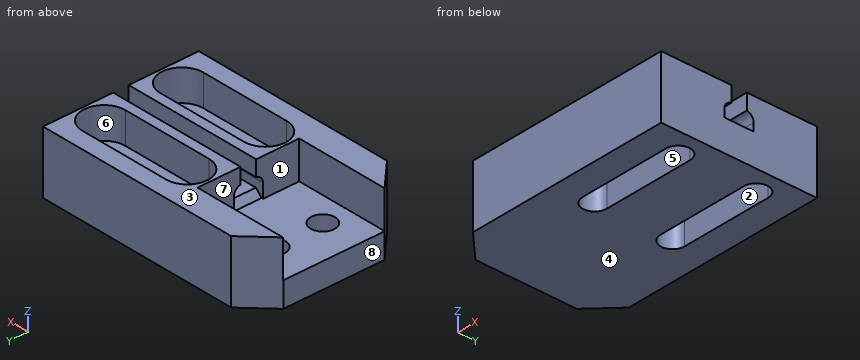
```python
from build123d import *

# Parameters (mm, degrees)
PROFILESKETCH3_W                           = 30
PROFILESKETCH3_H                           = 20
PROFILEBOSS_EXTRUDE1_DEPTH                 = 8
MICROSWITCHCUTSKETCH4_W                    = 12.05
MICROSWITCHCUTSKETCH4_H                    = 13.05
MICROSWITCHCUT_EXTRUDE1_DEPTH              = 4.8
SKETCH5_R                                  = 1.55
MICROSWITCHMOUNTINGHOLESCUT_EXTRUDE2_DEPTH = 3.1
SMALLCHANNELCABLESKETCH6_W                 = 17.95
SMALLCHANNELCABLESKETCH6_H                 = 2
SMALLCHANNELCABLECUT_EXTRUDE3_DEPTH        = 2
LARGECHANNELCABLESKETCH7_W                 = 17.95
LARGECHANNELCABLESKETCH7_H                 = 3.75
LARGECHANNELCABLECUT_EXTRUDE4_DEPTH        = 2
CHAMFER1_SIZE                              = 1
MOUNTSLOTBORECUT_EXTRUDE1_DEPTH            = 4
CHAMFER2_SIZE                              = 3.5
FILLET3_R                                  = 1


with BuildPart() as part:
    # ProfileSketch3 → ProfileBoss-Extrude1 (new body)
    with BuildSketch(Plane.XY):
        with Locations((15, 10)):
            Rectangle(PROFILESKETCH3_W, PROFILESKETCH3_H)
        with BuildLine():
            Line((15.15, 16.55), (26.9, 16.55))
            ThreePointArc((26.9, 16.55), (28.45, 15), (26.9, 13.45))
            Line((26.9, 13.45), (15.15, 13.45))
            ThreePointArc((15.15, 13.45), (13.6, 15), (15.15, 16.55))
        make_face(mode=Mode.SUBTRACT)
        with BuildLine():
            Line((15.15, 6.55), (26.9, 6.55))
            ThreePointArc((26.9, 6.55), (28.45, 5), (26.9, 3.45))
            Line((26.9, 3.45), (15.15, 3.45))
            ThreePointArc((15.15, 3.45), (13.6, 5), (15.15, 6.55))
        make_face(mode=Mode.SUBTRACT)
    extrude(amount=PROFILEBOSS_EXTRUDE1_DEPTH)

    # MicroSwitchCutSketch4 → MicroSwitchCut-Extrude1 (cut)
    with BuildSketch(Plane.XY.offset(8)):
        with Locations((6.025, 10)):
            Rectangle(MICROSWITCHCUTSKETCH4_W, MICROSWITCHCUTSKETCH4_H)
    extrude(amount=-MICROSWITCHCUT_EXTRUDE1_DEPTH, mode=Mode.SUBTRACT)

    # Sketch5 → MicroSwitchMountingHolesCut-Extrude2 (cut)
    with BuildSketch(Plane.XY.offset(3.2)):
        with Locations((5.05, 13.175)):
            Circle(SKETCH5_R)
        with Locations((5.05, 6.825)):
            Circle(SKETCH5_R)
    extrude(amount=-MICROSWITCHMOUNTINGHOLESCUT_EXTRUDE2_DEPTH, mode=Mode.SUBTRACT)

    # SmallChannelCableSketch6 → SmallChannelCableCut-Extrude3 (cut)
    with BuildSketch(Plane.XY.offset(8)):
        with Locations((21.025, 10)):
            Rectangle(SMALLCHANNELCABLESKETCH6_W, SMALLCHANNELCABLESKETCH6_H)
    extrude(amount=-SMALLCHANNELCABLECUT_EXTRUDE3_DEPTH, mode=Mode.SUBTRACT)

    # LargeChannelCableSketch7 → LargeChannelCableCut-Extrude4 (cut)
    with BuildSketch(Plane.XY.offset(6)):
        with Locations((21.025, 10)):
            Rectangle(LARGECHANNELCABLESKETCH7_W, LARGECHANNELCABLESKETCH7_H)
    extrude(amount=-LARGECHANNELCABLECUT_EXTRUDE4_DEPTH, mode=Mode.SUBTRACT)

    # Chamfer1
    # the kernel refuses this chamfer: 1 mm, written as the material it takes off along each edge
    with BuildSketch(Plane(origin=(12.05, 8.125, 4), x_dir=(0.9996219169112968, 0, 0.02749587661058651), z_dir=(0, 1, 0))) as chamfer1_piece_1_section:
        Polygon((CHAMFER1_SIZE * 0.999621916911, CHAMFER1_SIZE * 0.0274958766106), (-CHAMFER1_SIZE * 0.0274958766106, CHAMFER1_SIZE * 0.999621916911), (0, 0), align=None)
    chamfer1_piece_1 = extrude(amount=3.75, mode=Mode.PRIVATE)
    chamfer1_piece_1 = split(chamfer1_piece_1, bisect_by=Plane(origin=(12.395718412, 10, 3.2), z_dir=(0, 0, 1)), keep=Keep.TOP, mode=Mode.PRIVATE)
    add(chamfer1_piece_1, mode=Mode.SUBTRACT)

    # Sketch6 → MountSLotBoreCut-Extrude1 (cut)
    with BuildSketch(Plane.XY.offset(8)):
        with BuildLine():
            Line((15.15, 17.75), (26.9, 17.75))
            ThreePointArc((26.9, 17.75), (29.65, 15), (26.9, 12.25))
            Line((26.9, 12.25), (15.15, 12.25))
            ThreePointArc((15.15, 12.25), (12.4, 15), (15.15, 17.75))
        make_face()
        with BuildLine():
            Line((15.15, 7.75), (26.9, 7.75))
            ThreePointArc((26.9, 7.75), (29.65, 5), (26.9, 2.25))
            Line((26.9, 2.25), (15.15, 2.25))
            ThreePointArc((15.15, 2.25), (12.4, 5), (15.15, 7.75))
        make_face()
    extrude(amount=-MOUNTSLOTBORECUT_EXTRUDE1_DEPTH, mode=Mode.SUBTRACT)

    # Chamfer2
    chamfer2_edges = [part.edges().sort_by_distance(p)[0] for p in [
        (0, 20, 4),
        (0, 0, 4),
    ]]
    chamfer(chamfer2_edges, length=CHAMFER2_SIZE)

    # Fillet3
    # the kernel refuses this fillet: 1 mm, written as the material it adds along each edge
    with BuildSketch(Plane(origin=(12.05, 11.875, 6), x_dir=(0, 0, -1), z_dir=(1, 0, 0))) as fillet3_piece_1:
        with BuildLine():
            CenterArc((0.992156742, -1), FILLET3_R, 90, 82.819244219)
            Line((0, -0.875), (-0.019843135, -0.8725))
            ThreePointArc((-0.019843135, -0.8725), (-0.02, -0.4375), (-0.02, 0))
            Line((-0.02, 0), (0, 0.02))
            Line((0, 0.02), (0.992156742, 0.02))
            Line((0.992156742, 0.02), (0.992156742, 0))
        make_face()
    extrude(amount=17.95)
    with BuildSketch(Plane(origin=(30, 8.125, 6), x_dir=(0, 1, 0), z_dir=(-1, 0, 0))) as fillet3_piece_2:
        with BuildLine():
            CenterArc((1, 0.992156742), FILLET3_R, 180, 82.819244219)
            Line((0, 0.992156742), (-0.02, 0.992156742))
            Line((-0.02, 0.992156742), (-0.02, 0))
            Line((-0.02, 0), (0, -0.02))
            ThreePointArc((0, -0.02), (0.4375, -0.02), (0.8725, -0.019843135))
            Line((0.8725, -0.019843135), (0.875, 0))
        make_face()
    extrude(amount=17.95)


solid = part.part
```
Geometry check sheet. Reference: the model listing, model coordinates, mm. Face numbers are marked on the shaded views. A direction names the side the tool comes from. Coordinates: 2 decimals unless noted, no trailing zeros. Order: outer loops, then holes, each group sorted by start corner. A loop starts at its lowest first (then second) coordinate and runs counter-clockwise, first axis right, second up.
Q1. Depth check by flat-ended pin: pin 1 Ø4 at (y, z) = (11, 5) entering from -X; pin 2 Ø2.5 at (x, y) = (5.05, 13.175) entering from +Z; pin 3 Ø2.5 at (y, z) = (6, 5) entering from -X. Enter the tip coordinate at first touch or a pass-through.
Reply:
pin 1: stops at x = 0
pin 2: stops at z = 0.1
pin 3: stops at x = 12.05
Q2. Sectioned sample at D-D on z = 2.5. Record the cut outline in (x, y) (3 decimals).
Reply:
outline: (0, 3.5) - (3.5, 0) - (30, 0) - (30, 20) - (3.5, 20) - (0, 16.5) - close; hole circle Ø3.1 at (5.05, 6.825); hole circle Ø3.1 at (5.05, 13.175); hole (15.15, 3.45) - (26.9, 3.45) arc R1.55 ccw to (26.9, 6.55) - (15.15, 6.55) arc R1.55 ccw to start; hole (15.15, 13.45) - (26.9, 13.45) arc R1.55 ccw to (26.9, 16.55) - (15.15, 16.55) arc R1.55 ccw to start
Q3. Thickness scan on probe 1 along Y at (x, z) = (17.5, 1.5); probe 2 along Y at (x, z) = (5.05, 1.25) (3 decimals); probe 3 along X at (y, z) = (5, 3). Record the ranges inside material, lowest first.
Reply:
probe 1: y = 0 to 3.45, 6.55 to 13.45, 16.55 to 20
probe 2: y = 0 to 5.275, 8.375 to 11.625, 14.725 to 20
probe 3: x = 0 to 13.6, 28.45 to 30
Q4. Sectioned sample at A-A on x = 18. Record the cut outline in (y, z) (3 decimals).
Reply:
outline: (0, 0) - (3.45, 0) - (3.45, 4) - (2.25, 4) - (2.25, 8) - (0, 8) - close; (6.55, 0) - (13.45, 0) - (13.45, 4) - (12.25, 4) - (12.25, 8) - (11, 8) - (11, 6) arc R1 cw to (11.875, 5.008) - (11.875, 4) - (8.125, 4) - (8.125, 5.008) arc R1 cw to (9, 6) - (9, 8) - (7.75, 8) - (7.75, 4) - (6.55, 4) - close; (16.55, 0) - (20, 0) - (20, 8) - (17.75, 8) - (17.75, 4) - (16.55, 4) - close
Q5. Sectioned sample at C-C on x = 5.05. Record the cut outline in (y, z) (3 decimals), and give its area (3 significant figures).
Reply:
outline: (0, 0) - (20, 0) - (20, 8) - (16.525, 8) - (16.525, 3.2) - (14.725, 3.2) - (14.725, 0.1) - (11.625, 0.1) - (11.625, 3.2) - (8.375, 3.2) - (8.375, 0.1) - (5.275, 0.1) - (5.275, 3.2) - (3.475, 3.2) - (3.475, 8) - (0, 8) - close
area: 78.1 mm2
Q6. Tool access check on the marked faces 4, 5, 6, 7 and 8. Record the directions out of +Z, -Z, +X, -X, +Y, -Y that give a thin tool (end or side, any length) a straight path to the whole face; none if there is none.
Reply:
face 4: -Z, +X, -X, +Y, -Y
face 5: +Z, -Z
face 6: +Z
face 7: +Z, -X
face 8: +Z, -Z, -X, +Y, -Y
Q7. Draft check along X on the marked faces 1, 2 and 3. Enter one of: released by +X, released by -X, zero draft, split by the parting line, or undercut.
Reply:
face 1: released by -X
face 2: undercut
face 3: zero draft
Q8. Sectioned sample at B-B on y = 15.25. Record the cut outline in (x, z), and give its area (3 significant figures).
Reply:
outline: (0, 0) - (13.62, 0) - (13.62, 4) - (12.41, 4) - (12.41, 8) - (12.05, 8) - (12.05, 3.2) - (0, 3.2) - close; (28.43, 0) - (30, 0) - (30, 8) - (29.64, 8) - (29.64, 4) - (28.43, 4) - close
area: 54.0 mm2
